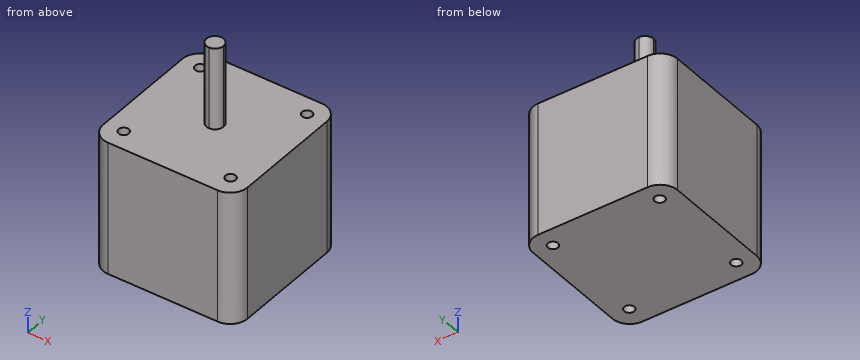
```python
from build123d import *

# Parameters (mm, degrees)
F0_W     = 42.3
F0_H     = 42.3
F1_DEPTH = 39
F2_R     = 5.08
F4_D     = 3
F6_DEPTH = 24


with BuildPart() as f1:
    # F0 (on Top) → F1 (new body)
    with BuildSketch(Plane.XY):
        with Locations((-0.275903, -1.519124)):
            Rectangle(F0_W, F0_H)
    extrude(amount=F1_DEPTH)

    # F2
    f2_edges = [f1.edges().sort_by_distance(p)[0] for p in [
        (20.874097, 19.630876, 19.5),
        (20.874097, -22.669124, 19.5),
        (-21.425903, 19.630876, 19.5),
        (-21.425903, -22.669124, 19.5),
    ]]
    fillet(f2_edges, radius=F2_R)

    # F4 (through all)
    with Locations(Plane.XY.offset(39)):
        with Locations((15.374097, 14.146936), (15.374097, -16.853064), (-15.925903, -16.853064), (-15.925903, 14.146936)):
            Hole(F4_D / 2)

    # F5 (on face) → F6 (join)
    with BuildSketch(Plane.XY.offset(39)):
        with BuildLine():
            ThreePointArc((-0.275903, -4.019124), (1.491864, -3.286891), (2.224097, -1.519124))
            Line((2.224097, -1.519124), (-0.275903, -1.519124))
            Line((-0.275903, -1.519124), (-0.275903, -4.019124))
        make_face()
        with BuildLine():
            Line((-0.275903, -1.519124), (2.224097, -1.519124))
            ThreePointArc((2.224097, -1.519124), (1.491864, 0.248643), (-0.275903, 0.980876))
            Line((-0.275903, 0.980876), (-0.275903, -1.519124))
        make_face()
        with BuildLine():
            Line((-0.275903, -4.019124), (-0.275903, -1.519124))
            Line((-0.275903, -1.519124), (-2.775903, -1.519124))
            ThreePointArc((-2.775903, -1.519124), (-2.04367, -3.286891), (-0.275903, -4.019124))
        make_face()
        with BuildLine():
            Line((-2.775903, -1.519124), (-0.275903, -1.519124))
            Line((-0.275903, -1.519124), (-0.275903, 0.980876))
            ThreePointArc((-0.275903, 0.980876), (-2.04367, 0.248643), (-2.775903, -1.519124))
        make_face()
    extrude(amount=F6_DEPTH)


solid = f1.part
```
CAD build for the part. Positions are in the model's coordinates, mm. Round coordinates to 2 decimals unless told otherwise and drop trailing zeros. Loops run counter-clockwise (first coordinate to the right, second up) from the corner with the lowest first, then second, coordinate; pieces in that order, holes last. Notation, with made-up numbers: M 57,45.25 L 115,45.25 A22 ccw 115,70.25 Z; hole C 63.5,-29 d11. An arc over 180 degrees is marked long. Return JSON: item names as keys, results as strings. Group by question number.
(1) Saw through at C-C, the plane y = -20. List the corners of the cut face in (x, z), and give its area (3 significant figures).
(2) Wall check: probe 1 along Z at (x, y) = (3.5, 13); probe 2 along Y at (x, z) = (0, 40); probe 3 along Y at (x, z) = (-2.5, 60). Give the ranges that are in metal, low to high. Write a range as [from, to].
(3) Saw through at D-D, the plane z = 59. List the corners of the cut face in (x, y), and give its area (3 significant figures).
(4) Saw through at A-A, the plane z = 7.5. List the corners of the cut face in (x, y).
(5) Saw through at B-B, the plane x = 0.5. List the corners of the cut face in (y, z), and give its area (3 significant figures).
(6) Drop a flat-ended pin along its axis: P1, Ø8, axis at x = 6.5, y = -10.5, coming from the +Z side. Give the stop position or say it passes through.
Answer list:
{
 "1": {"outline": "M -20.82,0 L 20.27,0 L 20.27,39 L -20.82,39 Z", "area": "1,600 mm2"},
 "2": {"probe 1": "[0, 39]", "probe 2": "[-4, 0.97]", "probe 3": "[-2.66, -0.38]"},
 "3": {"outline": "C -0.28,-1.52 d5", "area": "19.6 mm2"},
 "4": {"outline": "M -21.43,-17.59 A5.08 ccw -16.35,-22.67 L 15.79,-22.67 A5.08 ccw 20.87,-17.59 L 20.87,14.55 A5.08 ccw 15.79,19.63 L -16.35,19.63 A5.08 ccw -21.43,14.55 Z; hole C -15.93,-16.85 d3; hole C -15.93,14.15 d3; hole C 15.37,-16.85 d3; hole C 15.37,14.15 d3"},
 "5": {"outline": "M -22.67,0 L 19.63,0 L 19.63,39 L 0.86,39 L 0.86,63 L -3.9,63 L -3.9,39 L -22.67,39 Z", "area": "1,760 mm2"},
 "6": {"P1": "z = 39"}
}
